Source: CAD feature listing. Evaluate the final solid. Frame: model axes, mm. A direction names the side the tool comes from. Round coordinates to 2 decimals unless told otherwise and drop trailing zeros. Write each loop counter-clockwise with the first axis right and the second up, starting at its lowest first coordinate (ties: lowest second). Pieces come first, ordered by that corner, then holes.
```python
from build123d import *

# Parameters (mm, degrees)
F0_W          = 12.7
F0_H          = 25.4
F1_DEPTH      = 25.4
F3_DEPTH      = 12.701
F4_W          = 12.7
F4_H          = 19.128681
F5_DEPTH      = 12.7
F6_R          = 9.525
F7_DEPTH      = 6.35
F7_DEPTH_BACK = 19.05
F8_R          = 6.35
F9_DEPTH      = 25.401


with BuildPart() as f1:
    # F0 (on Top) → F1 (new body)
    with BuildSketch(Plane.XY):
        with Locations((-6.35, 12.7)):
            Rectangle(F0_W, F0_H)
    extrude(amount=F1_DEPTH)

    # F2 (on face) → F3 (cut, through all)
    with BuildSketch(Plane.YZ):
        Polygon((25.4, 19.05), (25.4, 25.4), (19.05, 25.4), align=None)
        Polygon((0, 25.4), (0, 19.05), (6.35, 25.4), align=None)
    extrude(amount=-F3_DEPTH, mode=Mode.SUBTRACT)

    # F4 (on face) → F5 (join)
    with BuildSketch(Plane.YZ):
        with Locations((12.7, 9.564341)):
            Rectangle(F4_W, F4_H)
    extrude(amount=F5_DEPTH)

    # F6 (on face) → F7 (join, two sides)
    with BuildSketch(Plane.XZ.offset(-6.35)) as f7_sk:
        with Locations((12.7, 9.56434)):
            Circle(F6_R)
    extrude(amount=F7_DEPTH)
    extrude(f7_sk.sketch, amount=-F7_DEPTH_BACK)

    # F8 (on face) → F9 (cut, through all)
    with BuildSketch(Plane.XZ):
        with Locations((12.7, 9.56434)):
            Circle(F8_R)
    extrude(amount=-F9_DEPTH, mode=Mode.SUBTRACT)


solid = f1.part
```
Q1. Section query C-C, the plane y = 16.5. Output: boundary loops of the cut face in (x, z) (3 decimals), and give its area (3 significant figures).
Q2. Section query B-B, the plane y = 3.25. Output: boundary loops of the cut face in (x, z) (3 decimals), and give its area (3 significant figures).
Q3. Section query D-D, the plane x = -7.5. Output: boundary loops of the cut face in (y, z).
Q4. Mould query, pull axis X, two halves, no side actions, for faces 4 (the face through (0, 13, 21)), 5 (the face through (-6, 25.4, 9)), 6 (the face through (-12.7, 13, 13)), 7 (the face through (8.02, 12.522, 13.856)). Classes: pulls with the +X half, pulls with the -X half, needs draft (parallel to the pull), parting line crosses it, or undercut.
Q5. Set-up query: faces 1 (the face through (2, 6.35, 9)), 2 (the face through (2, 19.05, 9)), 3 (the face through (6, 13, 19.129)). Return all of +Z, -Z, +X, -X, +Y, -Y with unobstructed straight access to the full face (end or side cutting, diameter ignored); none if empty.
Q6. Pin query (flat end, axial travel): P1, Ø10, axis at x = 12.7, z = 9.56, coming from the -Y side; P2, Ø4, axis at x = 3, z = 10.5, coming from the +Y side; P3, Ø4, axis at x = 16, y = 13.5, coming from the +Z side; P4, Ø4, axis at y = 8.5, z = 14, coming from the +X side. Return the tip coordinate at first contact, or that it passes through.
Q7. Line query: line 1 (Z direction, x = 12.7, y = 19); line 2 (X direction, y = 4, z = 5.5); line 3 (X direction, y = 23.75, z = 11.25). Output: solid intervals per line, ascending.
Q8. Section query A-A, the plane z = 8.5. Output: boundary loops of the cut face in (x, y).
Filled in:
1. outline: (-12.7, 0) - (12.7, 0) - (12.7, 0.039) arc R9.525 ccw to (12.7, 19.089) - (12.7, 19.129) - (0, 19.129) - (0, 25.4) - (-12.7, 25.4) - close; hole circle Ø12.7 at (12.7, 9.564)
1. area: 581 mm2
2. outline: (-12.7, 0) - (0, 0) - (0, 22.3) - (-12.7, 22.3) - close; circle Ø19.05 at (12.7, 9.564); hole circle Ø12.7 at (12.7, 9.564)
2. area: 442 mm2
3. outline: (0, 0) - (25.4, 0) - (25.4, 19.05) - (19.05, 25.4) - (6.35, 25.4) - (0, 19.05) - close
4. face 4: undercut
4. face 5: needs draft
4. face 6: pulls with the -X half
4. face 7: undercut
5. face 1: -Y
5. face 2: +Y
5. face 3: +Z, +X, +Y, -Y
6. P1: passes through
6. P2: stops at y = 25.4
6. P3: stops at z = 19
6. P4: stops at x = 21.91
7. line 1: z = 0.04 to 3.21, 15.91 to 19.09
7. line 2: x = -12.7 to 0, 4.09 to 7.82, 17.58 to 21.31
7. line 3: x = -12.7 to 0, 3.33 to 6.58, 18.82 to 22.07
8. outline: (-12.7, 0) - (0, 0) - (0, 6.35) - (3.23, 6.35) - (3.23, 0) - (6.44, 0) - (6.44, 25.4) - (3.23, 25.4) - (3.23, 19.05) - (0, 19.05) - (0, 25.4) - (-12.7, 25.4) - close; (18.96, 0) - (22.17, 0) - (22.17, 25.4) - (18.96, 25.4) - close
